Read the model definition and answer for the solid it produces. Units are mm, in the model's axes. A direction names the side the tool comes from. Coordinates: 2 decimals unless noted, no trailing zeros. Write each loop counter-clockwise with the first axis right and the second up, starting at its lowest first coordinate (ties: lowest second). Pieces come first, ordered by that corner, then holes. Notation, with made-up numbers: (87.25, 72.5) -> (129.25, 72.5) arc R22 cw to (129.25, 92.5) -> close; hole circle Ø5 at (0, 15). An arc over 180 degrees is marked (long way). Return JSON: item names as keys, results as strings.
from build123d import *

# Parameters (mm, degrees)
SKETCH1_R           = 28.9052
SKETCH1_R_2         = 2.8067
SKETCH1_R_3         = 18.7452
BOSS_EXTRUDE1_DEPTH = 12.954
SHELL1_T            = -2.54
FILLET1_R           = 2.54
WRAP1_START         = 2.54
WRAP1_DEPTH         = 6.35
WRAP1_2_DEPTH       = 1.13974359
WRAP1_START_2       = 4.900897436
WRAP1_3_DEPTH       = 1.13974359
CIRPATTERN3_COUNT   = 6


# Read off the part's stored shape, not the designer's step: Wrap1
with BuildPart() as part:
    # Sketch1 → Boss-Extrude1 (new body)
    with BuildSketch(Plane.XY):
        Circle(SKETCH1_R)
        with Locations((0, 23.8252)):
            Circle(SKETCH1_R_2, mode=Mode.SUBTRACT)
        with Locations((20.63322845, 11.9126)):
            Circle(SKETCH1_R_2, mode=Mode.SUBTRACT)
        with Locations((20.63322845, -11.9126)):
            Circle(SKETCH1_R_2, mode=Mode.SUBTRACT)
        with Locations((0, -23.8252)):
            Circle(SKETCH1_R_2, mode=Mode.SUBTRACT)
        with Locations((-20.63322845, -11.9126)):
            Circle(SKETCH1_R_2, mode=Mode.SUBTRACT)
        with Locations((-20.63322845, 11.9126)):
            Circle(SKETCH1_R_2, mode=Mode.SUBTRACT)
        Circle(SKETCH1_R_3, mode=Mode.SUBTRACT)
    extrude(amount=BOSS_EXTRUDE1_DEPTH)

    # Shell1
    shell1_openings = [part.faces().sort_by_distance(p)[0] for p in [
        (-28.087637483, 0, 12.954),
    ]]
    offset(amount=SHELL1_T, openings=shell1_openings)

    # Fillet1
    fillet1_edges = [part.edges().sort_by_distance(p)[0] for p in [
        (4.422660927, 20.820658236, 7.747),
        (-4.422660927, 20.820658236, 7.747),
        (4.927440918, 25.900658236, 7.747),
        (-4.927440918, 25.900658236, 7.747),
        (-20.242549419, 6.580192403, 7.747),
        (-15.819888492, 14.240465833, 7.747),
        (-24.894348466, 8.683040107, 7.747),
        (-19.966907548, 17.217618129, 7.747),
        (19.966907548, 17.217618129, 7.747),
        (24.894348466, 8.683040107, 7.747),
        (15.819888492, 14.240465833, 7.747),
        (20.242549419, 6.580192403, 7.747),
        (19.966907548, -17.217618129, 7.747),
        (24.894348466, -8.683040107, 7.747),
        (15.819888492, -14.240465833, 7.747),
        (20.242549419, -6.580192403, 7.747),
        (-4.927440918, -25.900658236, 7.747),
        (4.927440918, -25.900658236, 7.747),
        (-4.422660927, -20.820658236, 7.747),
        (4.422660927, -20.820658236, 7.747),
        (-15.819888492, -14.240465833, 7.747),
        (-20.242549419, -6.580192403, 7.747),
        (-19.966907548, -17.217618129, 7.747),
        (-24.894348466, -8.683040107, 7.747),
    ]]
    fillet(fillet1_edges, radius=FILLET1_R - 0.0001)  # a hair under: the kernel refuses the full size

    # Wrap1 outline → Wrap1 (cut)
    with BuildSketch(Plane.XY.offset(WRAP1_START)):
        with BuildLine():
            Line((-0.627114985, 27.628083644), (-0.655934608, 28.897756605))
            ThreePointArc((-0.655934608, 28.897756605), (-1.225495275, 28.879209622), (-1.79457962, 28.849437967))
            Line((-1.79457962, 28.849437967), (-1.715731658, 27.581887969))
            ThreePointArc((-1.715731658, 27.581887969), (-1.171651018, 27.610351554), (-0.627114985, 27.628083644))
        make_face()
    wrap1 = extrude(amount=WRAP1_DEPTH, mode=Mode.SUBTRACT)

    # Wrap1 2 outline → Wrap1 2 (cut)
    with BuildSketch(Plane.XY.offset(WRAP1_START)):
        with BuildLine():
            Line((1.240414833, 27.607347755), (1.297419192, 28.876067781))
            ThreePointArc((1.297419192, 28.876067781), (0.320925566, 28.903418376), (-0.655934608, 28.897756605))
            Line((-0.655934608, 28.897756605), (-0.627114985, 27.628083644))
            ThreePointArc((-0.627114985, 27.628083644), (0.306825146, 27.633496654), (1.240414833, 27.607347755))
        make_face()
    wrap1_2 = extrude(amount=WRAP1_2_DEPTH, mode=Mode.SUBTRACT)

    # Wrap1 3 outline → Wrap1 3 (cut)
    with BuildSketch(Plane.XY.offset(WRAP1_START_2)):
        with BuildLine():
            Line((1.240414833, 27.607347755), (1.297419192, 28.876067781))
            ThreePointArc((1.297419192, 28.876067781), (0.320925566, 28.903418376), (-0.655934608, 28.897756605))
            Line((-0.655934608, 28.897756605), (-0.627114985, 27.628083644))
            ThreePointArc((-0.627114985, 27.628083644), (0.306825146, 27.633496654), (1.240414833, 27.607347755))
        make_face()
    wrap1_3 = extrude(amount=WRAP1_3_DEPTH, mode=Mode.SUBTRACT)

    # CirPattern3: Wrap1, Wrap1 2, Wrap1 3 ×6 about axis
    cirpattern3_axis = Axis((0, 0, 0), (0, 0, 1))
    add([wrap1.rotate(cirpattern3_axis, i * 360 / CIRPATTERN3_COUNT) for i in range(1, CIRPATTERN3_COUNT)], mode=Mode.SUBTRACT)
    add([wrap1_2.rotate(cirpattern3_axis, i * 360 / CIRPATTERN3_COUNT) for i in range(1, CIRPATTERN3_COUNT)], mode=Mode.SUBTRACT)
    add([wrap1_3.rotate(cirpattern3_axis, i * 360 / CIRPATTERN3_COUNT) for i in range(1, CIRPATTERN3_COUNT)], mode=Mode.SUBTRACT)


solid = part.part
1. A tool of negligible diameter and unlimited length cuts with its end or side. For faces 4 (the face through (12, 20, 2.54)), 5 (the face through (0, -28, 2.54)), from which of +Z, -Z, +X, -X, +Y, -Y can it reach the whole face along a straight path? Write none if from no direction.
Taken from the geometry:
{"face 4": "+Z", "face 5": "-Y"}
2. For a pull along X with two mould halves and no side action, classify faces 1 (the face through (25, -13, 8.89)), 2 (the face through (-24, -15, 8.89)), 3 (the face through (-24.3, 14.4, 6.041)) as +X half, -X half, draft (parallel to the pull), parting line (faces both ways), or undercut.
Taken from the geometry:
{"face 1": "undercut", "face 2": "undercut", "face 3": "draft"}
3. Consider L1, parallel to Y at x = 0, z = 5; L2, parallel to Y at x = 0, z = 7; L3, parallel to Y at x = 21, z = 1.25. Determine where each line is inside the solid, lowest interval first.
Taken from the geometry:
{"L1": "y = -27.64 to -26.63, -21.02 to -18.75, 18.75 to 21.02, 26.63 to 27.64", "L2": "y = -28.91 to -26.63, -21.02 to -18.75, 18.75 to 21.02, 26.63 to 28.91", "L3": "y = -19.86 to -14.7, -9.13 to 9.13, 14.7 to 19.86"}
4. The part is cut by section A-A (y = 0). Determine the outline of the cut face in (x, z).
Taken from the geometry:
{"outline": "(-28.91, 0) -> (-18.75, 0) -> (-18.75, 12.95) -> (-21.29, 12.95) -> (-21.29, 2.54) -> (-26.37, 2.54) -> (-26.37, 12.95) -> (-28.91, 12.95) -> close; (18.75, 0) -> (28.91, 0) -> (28.91, 12.95) -> (26.37, 12.95) -> (26.37, 2.54) -> (21.29, 2.54) -> (21.29, 12.95) -> (18.75, 12.95) -> close"}
5. Flat-ended cylindrical pins translate along their axes: pin 1 Ø1 at (y, z) = (18.5, 3) entering from -X; pin 2 Ø1 at (x, z) = (-11.5, 6) entering from -Y; pin 3 Ø2 at (x, z) = (-19, 2) entering from +Y. Find the tip coordinate at first contact, or state that the pin passes through.
Taken from the geometry:
{"pin 1": "stops at x = -22.62", "pin 2": "stops at y = -26.73", "pin 3": "stops at y = 22.62"}
6. The part is cut by section B-B (z = 1). Determine the outline of the cut face in (x, y), then the cut area to 3 significant figures.
Taken from the geometry:
{"outline": "circle Ø57.81 at (0, 0); hole circle Ø5.61 at (-20.63, -11.91); hole circle Ø5.61 at (-20.63, 11.91); hole circle Ø37.49 at (0, 0); hole circle Ø5.61 at (0, -23.83); hole circle Ø5.61 at (0, 23.83); hole circle Ø5.61 at (20.63, -11.91); hole circle Ø5.61 at (20.63, 11.91)", "area": "1,370 mm2"}
